from build123d import *

# Parameters (mm, degrees)
F0_W     = 76.5
F0_H     = 76.5
F1_DEPTH = 0.795
F2_W     = 74.09
F2_H     = 74.09
F2_W_2   = 71.541
F2_H_2   = 71.684
F3_DEPTH = 3
F5_DEPTH = 0.795


with BuildPart() as f1:
    # F0 (on Front) → F1 (new body)
    with BuildSketch(Plane.XZ):
        with Locations((-38.25, 38.25)):
            Rectangle(F0_W, F0_H)
    extrude(amount=F1_DEPTH)

    # F2 (on face) → F3 (join)
    with BuildSketch(Plane.XZ.offset(0.795)):
        with Locations((-38.345, 38.345)):
            Rectangle(F2_W, F2_H)
        with Locations((-38.345, 38.345)):
            Rectangle(F2_W_2, F2_H_2, mode=Mode.SUBTRACT)
    extrude(amount=F3_DEPTH)

    # F4 (on face) → F5 (cut)
    with BuildSketch(Plane.XZ.offset(0.795)):
        Polygon((-72.97042, 0.726517), (-72.870188, -0.4949), (-1.538745, -0.4949), (-1.538745, 20.233245), (-20.977661, 20.233245), (-20.977661, 12.14023), (-7.426569, 12.14023), (-7.426569, 7.43499), (-33.211284, 7.43499), (-33.211284, 24.750275), (-2.344909, 24.750275), (-2.344909, 30.584774), (-44.315651, 30.584774), (-44.315651, 7.43499), (-72.547097, 7.43499), (-72.547097, 30.584774), (-52.408666, 30.584774), (-52.408666, 15.339793), (-57.490327, 15.339793), (-57.490327, 27.197001), (-65.771547, 27.197001), (-65.771547, 12.14023), (-48.079845, 12.14023), (-48.079845, 33.784337), (-72.735306, 33.784337), (-72.735306, 38.677789), (-44.503864, 38.677789), (-44.503864, 33.784337), (-2.344909, 33.784337), (-2.344909, 43.571237), (-72.735306, 43.571237), (-72.735306, 49.970365), (-2.344909, 49.970365), (-2.344909, 62.768615), (-11.75539, 62.768615), (-11.75539, 54.675604), (-23.424385, 54.675604), (-23.424385, 58.628007), (-16.46063, 58.628007), (-16.46063, 62.956824), (-30.011721, 62.956824), (-30.011721, 55.052026), (-72.735306, 55.052026), (-72.735306, 62.956824), (-65.771547, 62.956824), (-65.771547, 59.945471), (-34.905173, 59.945471), (-34.905173, 65.591767), (-2.344909, 65.591767), (-2.344909, 72.555519), (-72.735306, 72.555519), (-72.735306, 69.732375), (-38.104736, 69.732375), (-38.104736, 62.956824), (-44.880282, 62.956824), (-44.880282, 66.156394), (-72.735306, 66.156394), (-72.735306, 65.211832), (-46.141766, 65.211832), (-46.141766, 62.145642), (-37.366107, 62.145642), (-37.366107, 70.498376), (-71.728628, 70.498376), (-71.728628, 71.661412), (-3.320788, 71.661412), (-3.320788, 66.156394), (-36.097341, 66.156394), (-36.097341, 60.77114), (-64.961855, 60.77114), (-64.961855, 63.837334), (-73.843245, 63.837334), (-73.843245, 54.215829), (-28.907644, 54.215829), (-28.907644, 62.039911), (-17.488717, 62.039911), (-17.488717, 59.50237), (-24.57268, 59.50237), (-24.57268, 53.898636), (-10.510482, 53.898636), (-10.510482, 61.511255), (-3.320788, 61.511255), (-3.320788, 51.043905), (-73.948969, 51.043905), (-73.948969, 42.69117), (-3.320788, 42.69117), (-3.320788, 34.65563), (-43.604229, 34.65563), (-43.604229, 39.624977), (-73.948969, 39.624977), (-73.948969, 32.858203), (-49.20796, 32.858203), (-49.20796, 13.278713), (-64.569082, 13.278713), (-64.569082, 26.011829), (-58.600437, 26.011829), (-58.600437, 14.605078), (-51.305421, 14.605078), (-51.305421, 31.715206), (-73.948969, 31.715206), (-73.948969, 6.514244), (-43.081951, 6.514244), (-43.081951, 29.327746), (-3.320788, 29.327746), (-3.320788, 25.879192), (-34.905173, 25.879192), (-34.905173, 6.779518), (-5.943694, 6.779518), (-5.943694, 13.278713), (-19.87054, 13.278713), (-19.87054, 19.247362), (-2.673007, 19.247362), (-2.673007, 0.726517), align=None)
    extrude(amount=-F5_DEPTH, mode=Mode.SUBTRACT)


solid = f1.part
Can you work these out from the model? Positions are in its coordinate system, mm. A direction names the side the tool comes from. Coordinates: 2 decimals unless noted, no trailing zeros. Write each loop counter-clockwise with the first axis right and the second up, starting at its lowest first coordinate (ties: lowest second). Pieces come first, ordered by that corner, then holes. Notation, with made-up numbers: (86.25, -10) -> (111.25, -10) arc R19 cw to (111.25, 14) -> close; hole circle Ø3 at (-17.5, 35.5). An arc over 180 degrees is marked (long way). Answer as CSV lines item,"result".
1) Will these pins go through, and if not, where does the flat tip stop? P1, Ø3, axis at x = -31.5, z = 46, coming from the -Y side (3 decimals); P2, Ø6, axis at x = -16, z = 63, coming from the +Y side; P3, Ø0.9, axis at x = -58.5, y = -0.5, coming from the -Z side; P4, Ø1.5, axis at y = -3, z = 36.5, coming from the -X side.
Check result:
P1,"y = -0.795"
P2,"y = 0"
P3,"z = 0.73"
P4,"x = -75.39"
2) If I drill on line 1 (X direction, y = -0.25, z = 55.5); line 2 (Z direction, x = -49.5, y = -3.2); line 3 (X direction, y = -1.05, z = 27.5), over which ranges is the centre line in solid material (lowest first)? Write a range as from..to.
Check result:
line 1,"-76.5..-73.84, -72.74..-30.01, -28.91..-24.57, -23.42..-11.76, -10.51..-3.32, -2.34..0"
line 2,"1.3..2.5, 74.19..75.39"
line 3,"-75.39..-74.12, -2.57..-1.3"
3) If we section it at A-A on z = 9: Count the separate pieces of the cut face and the enclosed holes in it, then the cut area to 3 significant figures.
Check result:
separate pieces,"6"
enclosed holes,"0"
area,"62.9 mm²"
4) If we mould it in two halves opening along X, with no side actions, what happens to faces 5 (the flat face through (-39, -2, 75.39)), 6 (the flat face through (-1.3, -2, 38)), 7 (the flat face through (-38, -0.795, 47))? For each: +X half, -X half, draft (parallel to the pull), parting line (faces both ways), or undercut.
Check result:
face 5,"draft"
face 6,"+X half"
face 7,"undercut"
5) On a 3-axis mill with a long thin cutter (end or side, diameter ignored), from which of +Z, -Z, +X, -X, +Y, -Y can I reach the whole of each face in a straight line? I mean faces 1 (the flat face through (-39, -2, 1.3)), 2 (the flat face through (-54, -0.795, 23)), 3 (the flat face through (-75.39, -2, 38)), 4 (the flat face through (-39, 0, 39)). Say none if no direction works.
Check result:
face 1,"-Z, +X, -X, -Y"
face 2,"-Y"
face 3,"+Z, -Z, -X, -Y"
face 4,"+Z, -Z, +X, -X, +Y"
6) If we section it at B-B on y = -2.15: Please give me the cut outline in (x, z), then the cut area to 3 significant figures.
Check result:
outline,"(-75.39, 1.3) -> (-1.3, 1.3) -> (-1.3, 75.39) -> (-75.39, 75.39) -> close; hole (-74.12, 2.5) -> (-2.57, 2.5) -> (-2.57, 74.19) -> (-74.12, 74.19) -> close"
area,"361 mm²"
